from build123d import *

# Parameters (mm, degrees)
EXTRUDE_1_DEPTH     = 18
SKETCH_2_R          = 13.25
CUT_EXTRUDE_1_DEPTH = 76.986840966
FILLET_1_R          = 1.5


with BuildPart() as part:
    # ｽｹｯﾁ1 → ﾎﾞｽ - 押し出し1 (new body)
    with BuildSketch(Plane.XY):
        Polygon((0, 0), (0, 14.5), (15, 14.5), (15, 50.5), (0, 50.5), (0, 65), (35, 65), (35, 0), align=None)
    extrude(amount=EXTRUDE_1_DEPTH)

    # ｽｹｯﾁ2 → ｶｯﾄ - 押し出し1 (cut, through all)
    with BuildSketch(Plane.ZY):
        with Locations((0, 32.5)):
            Circle(SKETCH_2_R)
    extrude(amount=-CUT_EXTRUDE_1_DEPTH, mode=Mode.SUBTRACT)

    # ﾌｨﾚｯﾄ1
    fillet_1_edges = [part.edges().sort_by_distance(p)[0] for p in [
        (0, 57.75, 0),
        (17.5, 65, 0),
        (7.5, 14.5, 18),
        (35, 55.375, 0),
        (17.5, 0, 0),
        (0, 7.25, 0),
        (7.5, 14.5, 0),
        (15, 16.875, 0),
        (0, 7.25, 18),
        (17.5, 0, 18),
        (35, 32.5, 18),
        (15, 48.125, 0),
        (35, 9.625, 0),
        (25, 19.25, 0),
        (25, 45.75, 0),
        (17.5, 65, 18),
        (15, 32.5, 13.25),
        (0, 57.75, 18),
        (7.5, 50.5, 18),
        (15, 32.5, 18),
        (7.5, 50.5, 0),
    ]]
    fillet(fillet_1_edges, radius=FILLET_1_R)


solid = part.part
Geometry check sheet. Reference: the model listing, model coordinates, mm. A direction names the side the tool comes from. Round coordinates to 2 decimals unless told otherwise and drop trailing zeros. Order: outer loops, then holes, each group sorted by start corner. A loop starts at its lowest first (then second) coordinate and runs counter-clockwise, first axis right, second up. Notation, with made-up numbers: M -29.75,30.25 L 15.25,30.25 A12 cw 15.25,44.25 Z; hole C 51.5,38 d6. An arc over 180 degrees is marked long. Answer in a Markdown table with one row per item.
(1) Draft check along Y on faces 5 (the face through (0.43, 7.35, 0.45)), 6 (the face through (25.62, 32.228, 13.247)), 7 (the face through (17.26, 0.45, 0.43)). Enter one of: released by +Y, released by -Y, zero draft, split by the parting line, or undercut.
Responses:
| item | result |
|---|---|
| face 5 | zero draft |
| face 6 | undercut |
| face 7 | released by -Y |
(2) Tool access check on faces 1 (the face through (7, 14.5, 9)), 2 (the face through (8.37, 14.05, 17.57)), 3 (the face through (8.13, 50.95, 0.43)), 4 (the face through (18, 0, 9)). Record the directions out of +Z, -Z, +X, -X, +Y, -Y that give a thin tool (end or side, any length) a straight path to the whole face; none if there is none.
Responses:
| item | result |
|---|---|
| face 1 | +Z, -Z, -X |
| face 2 | +Z, -X |
| face 3 | -Z, -X |
| face 4 | +Z, -Z, +X, -X, -Y |
(3) Sectioned sample at B-B, the plane z = 15.5. Record the cut outline in (x, y).
Responses:
| item | result |
|---|---|
| outline | M 0,0 L 35,0 L 35,65 L 0,65 L 0,50.5 L 15,50.5 L 15,14.5 L 0,14.5 Z |
(4) Sectioned sample at C-C, the plane x = 32. Record the cut outline in (y, z).
Responses:
| item | result |
|---|---|
| outline | M 0,1.5 A1.5 ccw 1.5,0 L 17.83,0 A1.5 ccw 19.32,1.35 A13.25 cw 45.68,1.35 A1.5 ccw 47.17,0 L 63.5,0 A1.5 ccw 65,1.5 L 65,16.5 A1.5 ccw 63.5,18 L 1.5,18 A1.5 ccw 0,16.5 Z |
(5) Sectioned sample at A-A, the plane x = 6. Record the cut outline in (y, z), and give its area (3 significant figures).
Responses:
| item | result |
|---|---|
| outline | M 0,1.5 A1.5 ccw 1.5,0 L 13,0 A1.5 ccw 14.5,1.5 L 14.5,16.5 A1.5 ccw 13,18 L 1.5,18 A1.5 ccw 0,16.5 Z; M 50.5,1.5 A1.5 ccw 52,0 L 63.5,0 A1.5 ccw 65,1.5 L 65,16.5 A1.5 ccw 63.5,18 L 52,18 A1.5 ccw 50.5,16.5 Z |
| area | 518 mm² |
(6) Scan lines: probe 1 along Y at (x, z) = (8, 6.25); probe 2 along X at (y, z) = (43.5, 12.25); probe 3 along Y at (x, z) = (21.5, 10.75). Record each from-to range of solid material in increasing order. Write a range as from..to.
Responses:
| item | result |
|---|---|
| probe 1 | y = 0..14.5, 50.5..65 |
| probe 2 | x = 15..35 |
| probe 3 | y = 0..24.75, 40.25..65 |
